from build123d import *

# Parameters (mm, degrees)
F1_DEPTH = 9.525
F2_R     = 5.2336589489
F3_DEPTH = 25.4


with BuildPart() as f1:
    # F0 (on Top) → F1 (new body)
    with BuildSketch(Plane.XY):
        with BuildLine():
            Line((7.7218987456, 12.310102582), (7.62, 12.310102582))
            Line((7.62, 12.310102582), (7.62, 22.225))
            Line((7.62, 22.225), (-7.62, 22.225))
            Line((-7.62, 22.225), (-7.62, 9.525))
            Line((-7.62, 9.525), (-19.05, 9.525))
            Line((-19.05, 9.525), (-19.05, 0))
            Line((-19.05, 0), (-19.05, -9.525))
            Line((-19.05, -9.525), (-7.62, -9.525))
            Line((-7.62, -9.525), (-7.62, -22.225))
            Line((-7.62, -22.225), (7.62, -22.225))
            Line((7.62, -22.225), (7.62, -12.310102582))
            Line((7.62, -12.310102582), (7.7218987456, -12.310102582))
            ThreePointArc((7.7218987456, -12.310102582), (9.0713316669, -8.995991319), (12.3745044693, -7.62))
            Line((12.3745044693, -7.62), (76.2223307455, -7.62))
            ThreePointArc((76.2223307455, -7.62), (89.0032784798, -8.6995142786), (101.4220945716, -11.907470472))
            add(Edge.make_bspline(
                [(101.4220945716, -11.907470472), (108.8479078103, -14.5096420416), (115.4579135782, -16.9617020129), (119.7392494006, -18.9785115521)],
                knots=[0.2329982419, 0.2329982419, 0.2329982419, 0.2329982419, 0.665918316, 0.665918316, 0.665918316, 0.665918316], degree=3))
            ThreePointArc((119.7392494006, -18.9785115521), (124.4257242361, -20.1562770444), (129.2577777778, -20.1941783568))
            ThreePointArc((129.2577777778, -20.1941783568), (131.0404681386, -20.6690128346), (132.0316072031, -22.225))
            Line((132.0316072031, -22.225), (147.32, -22.225))
            Line((147.32, -22.225), (147.32, -11.1125))
            Line((147.32, -11.1125), (158.75, 0))
            Line((158.75, 0), (147.32, 11.1125))
            Line((147.32, 11.1125), (147.32, 22.225))
            Line((147.32, 22.225), (132.08, 22.225))
            Line((132.08, 22.225), (132.08, 22.7184506514))
            ThreePointArc((132.08, 22.7184506514), (131.2333333333, 20.8252464304), (129.2577777778, 20.1941783568))
            ThreePointArc((129.2577777778, 20.1941783568), (124.4257242361, 20.1562770444), (119.7392494006, 18.9785115521))
            add(Edge.make_bspline(
                [(101.4220945716, 11.907470472), (108.8479078103, 14.5096420416), (115.4579135782, 16.9617020129), (119.7392494006, 18.9785115521)],
                knots=[0.2329982419, 0.2329982419, 0.2329982419, 0.2329982419, 0.665918316, 0.665918316, 0.665918316, 0.665918316], degree=3))
            ThreePointArc((101.4220945716, 11.907470472), (89.0032784798, 8.6995142786), (76.2223307455, 7.62))
            Line((76.2223307455, 7.62), (12.3745044693, 7.62))
            ThreePointArc((12.3745044693, 7.62), (9.0713316669, 8.995991319), (7.7218987456, 12.310102582))
        make_face()
        with BuildLine():
            ThreePointArc((114.3, 0), (127, 12.7), (139.7, 0))
            ThreePointArc((139.7, 0), (127, -12.7), (114.3, 0))
        make_face(mode=Mode.SUBTRACT)
    extrude(amount=F1_DEPTH)

    # F2 (on face) → F3 (cut)
    with BuildSketch(Plane.XZ.offset(9.525)):
        with Locations((-19.05, 9.525)):
            Circle(F2_R)
    extrude(amount=-F3_DEPTH, mode=Mode.SUBTRACT)


solid = f1.part
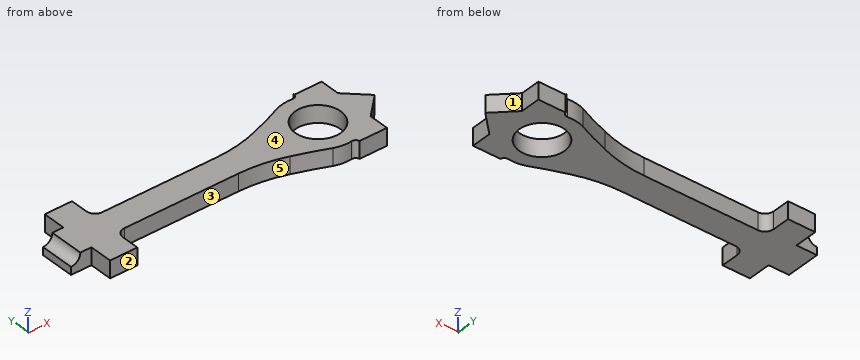
Check sheet for the modelled part. Datum: model origin and axes. Units: mm. Face numbers are marked on the shaded views. A direction names the side the tool comes from. Round coordinates to 2 decimals unless told otherwise and drop trailing zeros. Order: outer loops, then holes, each group sorted by start corner. A loop starts at its lowest first (then second) coordinate and runs counter-clockwise, first axis right, second up. Notation, with made-up numbers: M -20.75,37 L 38.25,37 A13 ccw 38.25,48 Z; hole C 47.25,33.5 d11. An arc over 180 degrees is marked long. One line per item, written item: value. Start each with the question number.
1. Section check B-B on y = 5. Enter the section's corners in (x, z) (3 decimals), and give its area (3 significant figures).
2. Release check for a two-part mould opening along X. For the marked faces 1, 2 and 3 record: released by +X, released by -X, zero draft, split by the parting line, or undercut.
3. Section check A-A on x = 127. Enter the section's corners in (y, z) (3 decimals).
4. Scan lines: line 1 along Y through (x, z) = (127, 3.5); line 2 along X through (y, z) = (17.5, 4.5); line 3 along X through (y, z) = (1, 5). Record each from-to range of solid material in increasing order.
5. Gauge pin test, flat ends, axial feed: P1, Ø1.5, axis at x = 130.5, z = 5.5, coming from the +Y side; P2, Ø3, axis at y = 15, z = 5, coming from the +X side; P3, Ø1.5, axis at x = 124, z = 3.5, coming from the +Y side; P4, Ø20.5, axis at x = 127, y = 0, coming from the -Z side. Record the tip position at first contact, or that the pin passes through.
6. Access from +Z, -Z, +X, -X, +Y, -Y to the whole of each face (thin tool, end or side, straight path). Record for the marked faces 4 and 5.
Results found:
1. outline: M -19.05,0 L 115.326,0 L 115.326,9.525 L -13.816,9.525 A5.234 cw -19.05,4.291 Z; M 138.674,0 L 153.607,0 L 153.607,9.525 L 138.674,9.525 Z
1. area: 1,400 mm^2
2. face 1: released by +X
2. face 2: zero draft
2. face 3: undercut
3. outline: M -20.32,0 L -12.7,0 L -12.7,9.525 L -20.32,9.525 Z; M 12.7,0 L 20.32,0 L 20.32,9.525 L 12.7,9.525 Z
4. line 1: -20.32 to -12.7, 12.7 to 20.32
4. line 2: -7.62 to 7.62, 116.38 to 147.32
4. line 3: -16.42 to 114.34, 139.66 to 157.72
5. P1: y = 20.84
5. P2: x = 147.32
5. P3: y = 20.2
5. P4: through
6. face 4: +Z, +X, -X, +Y, -Y
6. face 5: +Z, -Z, -Y
